Autodesk Inventor part; units mm, degrees
ref_plane "Start plane" through (0, 0, 0) normal (0, 0, 1) x (1, 0, 0)
ref_plane "End plane" through (0, 0, 561.975) normal (0, 0, 1) x (1, 0, 0)
ref_plane "Work Plane4" through (19.05, 0, 0) normal (0, 0.7071, -0.7071) x (1, 0, 0)
ref_plane "Start plane" through (0, 0, 0) normal (0, 0, 1) x (1, 0, 0)
ref_plane "End plane" through (0, 0, 561.975) normal (0, 0, 1) x (1, 0, 0)
sketch "Sketch" plane through (0, 0, 0) normal (0, 0, 1) x (1, 0, 0)
  line L0 (38.1, 0) -> (0, 0)
  line L1 (0, 0) -> (0, 38.1)
  line L2 (0, 38.1) -> (2.4765, 38.1)
  line L3 (4.7625, 35.814) -> (4.7625, 9.5885)
  line L4 (9.5885, 4.7625) -> (35.814, 4.7625)
  line L5 (38.1, 2.4765) -> (38.1, 0)
  line L6 (0, -11.0414) -> (0, 31.5385) construction
  line L7 (-11.0414, 0) -> (31.5385, 0) construction
  arc A0 (4.7625, 9.5885) -> (9.5885, 4.7625) centre (9.5885, 9.5885) ccw
  arc A1 (4.7625, 35.814) -> (2.4765, 38.1) centre (2.4765, 35.814) ccw
  arc A2 (38.1, 2.4765) -> (35.814, 4.7625) centre (35.814, 2.4765) ccw
  line L8 (0, 48.4964) -> (0, -20.9644) construction
  line L9 (-20.9644, 0) -> (48.4964, 0) construction
  point P0 (4.7625, 38.1)
  point P1 (4.7625, 4.7625)
  point P2 (38.1, 4.7625)
  dimension "d0" = 38.1
  dimension "d1" = 38.1
  dimension "d2" = 4.7625
  dimension "d3" = 4.7625
  dimension "d10" = 0
  dimension "d11" = 0
  dimension "d14" = 4.826
  dimension "d15" = 2.286
extrude "Body" add sketch "Sketch" along normal up to surface (561.975 mm away) from surface at 0
sketch "Sketch3" plane through (0, 0, 0) normal (0, 0, 1) x (1, 0, 0)
  line L0 (0, 0) -> (10, 0)
ref_plane "Work Plane3" through (0, 0, 0) normal (0, -1, 0) x (1, 0, 0)
sketch "Sketch4" plane through (0, 0, 0) normal (0, -1, 0) x (1, 0, 0)
  line L0 (-2, 0) -> (12, 0)
  line L1 (-2, 561.975) -> (12, 561.975)
  dimension "d17" = 561.975
ref_plane "Work Plane4" through (19.05, 0, 0) normal (0, 0.7071, -0.7071) x (1, 0, 0)
split "Split1" plane through (19.05, 0, 0) removes the side toward (0, 0.7071, -0.7071)
ref_plane "Work Plane5" through (19.05, 0, 561.975) normal (0, 0.7071, 0.7071) x (1, 0, 0)
split "Split2" plane through (19.05, 0, 561.975) removes the side toward (0, 0.7071, 0.7071)
equation "\"d0\" = G_H"
equation "\"d1\" = G_H"
equation "\"d2\" = G_T"
equation "\"d3\" = G_T"
equation "\"d14\" = G_IR"
equation "\"d15\" = G_ER"
equation "\"d4\" = G_L"
equation "\"G_H\" = 38.1"
equation "\"G_T\" = 4.7625"
equation "\"G_ER\" = 2.286"
equation "\"G_IR\" = 4.826"
equation "\"G_L\" = d17"
equation "\"ex\" = 0"
equation "\"G_OFFSET_START\" = 0"
equation "\"G_OFFSET_END\" = 0"
equation "\"d13\" = G_OFFSET_END + B_L"
equation "\"B_L\" = 561.975"
properties part number "AISC - L 1.5 x 1.5 x 3/16 - 22.125" material "Aluminum 6061-AHC"
Input: part model. Units: mm. Frame: model coordinates. A direction names the side the tool comes from. Round coordinates to 2 decimals unless told otherwise and drop trailing zeros. Loops run counter-clockwise (first coordinate to the right, second up) from the corner with the lowest first, then second, coordinate; pieces in that order, holes last.
1) Section query A-A on z = 285.5. Return the cut outline in (x, y), plus the area to 3 significant figures.
Ans:
outline: (0, 0) - (38.1, 0) - (38.1, 2.48) arc R2.29 ccw to (35.81, 4.76) - (9.59, 4.76) arc R4.83 cw to (4.76, 9.59) - (4.76, 35.81) arc R2.29 ccw to (2.48, 38.1) - (0, 38.1) - close
area: 343 mm2
2) Set-up query: faces 1 (the flat face through (0, 19, 277)), 2 (the flat face through (4.762, 23, 277)). Return all of +Z, -Z, +X, -X, +Y, -Y with unobstructed straight access to the full face (end or side cutting, diameter ignored); none if empty.
Ans:
face 1: +Z, -Z, -X, +Y, -Y
face 2: +Z, -Z, +X, +Y
3) Material intervals for line 1 (X direction, y = 18, z = 273.5); line 2 (Y direction, x = 4, z = 193), sorted ascending.
Ans:
line 1: x = 0 to 4.76
line 2: y = 0 to 37.52
4) Section query B-B on x = 31. Return the cut outline in (y, z) (1 decimal), plus the area to 3 significant figures.
Ans:
outline: (0, 0) - (4.8, 4.8) - (4.8, 557.2) - (0, 562) - close
area: 2,650 mm2
5) Pin query (flat end, axial travel): pin 1 (13 mm diameter, centred on x = 21.5, z = 384.5, fed in from +Y); pin 2 (8 mm diameter, centred on y = 18.5, z = 264.5, fed in from +X). Return the tip coordinate at first contact, or that it passes through.
Ans:
pin 1: stops at y = 4.76
pin 2: stops at x = 4.76
6) Section query C-C on y = 20.5. Return the cut outline in (x, z) (1 decimal), plus the area to 3 significant figures.
Ans:
outline: (0, 20.5) - (4.8, 20.5) - (4.8, 541.5) - (0, 541.5) - close
area: 2,480 mm2
